CAD build for the part. Positions are in the model's coordinates, mm. Face numbers are marked on the shaded views. A direction names the side the tool comes from. Give positions to 0.01 mm unless a question says otherwise; leave off trailing zeros. Write each loop counter-clockwise with the first axis right and the second up, starting at its lowest first coordinate (ties: lowest second). Pieces come first, ordered by that corner, then holes. Notation, with made-up numbers: M 43,9 L 50,9 A27 cw 50,38 Z; hole C 78,23.25 d8. An arc over 180 degrees is marked long. One line per question, with ' | ' between items. Start each with the question number.
1. Cut at B-B, the plane z = -9.75. Write the cut outline in (x, y), then the cut area to 3 significant figures.
2. Wall check: L1, parallel to X at y = 1, z = 6.5; L2, parallel to Y at x = 7.5, z = 10.5; L3, parallel to Z at x = 11, y = 0.9. Give the ranges that are in metal, low to high.
3. Cut at C-C, the plane y = 1.55. Write the cut outline in (x, z), then the cut area to 3 significant figures.
4. Flat gauge pins, fed straight in: pin 1 (0.6 mm diameter, centred on x = 11, y = 1.5, fed in from +Z); pin 2 (5 mm diameter, centred on x = 1.5, z = -0.5, fed in from +Y). Where does each tip first touch, or does it go through?
5. Cut at D-D, the plane x = -8. Write the cut outline in (y, z).
6. Which spindle directions (+Z, -Z, +X, -X, +Y, -Y) get a long thin tool onto all of the face, cutting with end or side? Do the marked faces 1 and 2. Say none if no direction does.
7. Cut at A-A, the plane x = 11.25. Write the cut outline in (y, z).
```python
from build123d import *

# Parameters (mm, degrees)
SKETCH1_W           = 26
SKETCH1_H           = 24
BOSS_EXTRUDE1_DEPTH = 0.7
SKETCH2_W           = 2
SKETCH2_H           = 22
BOSS_EXTRUDE2_DEPTH = 1.3
CUT_EXTRUDE2_DEPTH  = 0.4
CUT_EXTRUDE3_DEPTH  = 0.4
SKETCH4_W           = 1
SKETCH4_H           = 24
BOSS_EXTRUDE3_DEPTH = 0.7
CUT_EXTRUDE4_DEPTH  = 0.4


with BuildPart() as part:
    # Sketch1 → Boss-Extrude1 (new body)
    with BuildSketch(Plane(origin=(0, 0, 0), x_dir=(1, 0, 0), z_dir=(0, 1, 0))):
        Rectangle(SKETCH1_W, SKETCH1_H)
    extrude(amount=BOSS_EXTRUDE1_DEPTH)

    # Sketch2 → Boss-Extrude2 (add)
    with BuildSketch(Plane(origin=(0, 0.7, 0), x_dir=(1, 0, 0), z_dir=(0, 1, 0))):
        with Locations((11, 0)):
            Rectangle(SKETCH2_W, SKETCH2_H)
    extrude(amount=BOSS_EXTRUDE2_DEPTH)

    # Sketch3 → Cut-Extrude2 (cut)
    with BuildSketch(Plane(origin=(0, 0.7, 0), x_dir=(1, 0, 0), z_dir=(0, 1, 0))):
        with BuildLine():
            Line((-2.366025404, 7.5), (-11.026279442, -7.5))
            ThreePointArc((-11.026279442, -7.5), (-11.026279442, -8.5), (-10.160254038, -9))
            Line((-10.160254038, -9), (7.160254038, -9))
            ThreePointArc((7.160254038, -9), (8.026279442, -8.5), (8.026279442, -7.5))
            Line((8.026279442, -7.5), (-0.633974596, 7.5))
            ThreePointArc((-0.633974596, 7.5), (-1.5, 8), (-2.366025404, 7.5))
        make_face()
        Polygon((7.160254038, -8), (-1.5, 7), (-10.160254038, -8), align=None, mode=Mode.SUBTRACT)
    extrude(amount=-CUT_EXTRUDE2_DEPTH, mode=Mode.SUBTRACT)

    # Sketch5 → Cut-Extrude3 (cut)
    with BuildSketch(Plane(origin=(0, 0.7, 0), x_dir=(1, 0, 0), z_dir=(0, 1, 0))):
        with BuildLine():
            Line((-4.151650429, -6.00520382), (-2.369048338, -4.222601728))
            ThreePointArc((-2.369048338, -4.222601728), (-2.33335535, -4.247204418), (-2.296966313, -4.270765398))
            Line((-2.296966313, -4.270765398), (-2.756186431, -5.379420837))
            Line((-2.756186431, -5.379420837), (-2.294246665, -5.570762553))
            Line((-2.294246665, -5.570762553), (-1.835026546, -4.462107114))
            ThreePointArc((-1.835026546, -4.462107114), (-1.792635483, -4.471177921), (-1.75, -4.479019946))
            Line((-1.75, -4.479019946), (-1.75, -7))
            Line((-1.75, -7), (-1.25, -7))
            Line((-1.25, -7), (-1.25, -4.479019946))
            ThreePointArc((-1.25, -4.479019946), (-1.207364517, -4.471177921), (-1.164973454, -4.462107114))
            Line((-1.164973454, -4.462107114), (-0.705753335, -5.570762553))
            Line((-0.705753335, -5.570762553), (-0.243813569, -5.379420837))
            Line((-0.243813569, -5.379420837), (-0.703033687, -4.270765398))
            ThreePointArc((-0.703033687, -4.270765398), (-0.66664465, -4.247204418), (-0.630951662, -4.222601728))
            Line((-0.630951662, -4.222601728), (1.151650429, -6.00520382))
            Line((1.151650429, -6.00520382), (1.50520382, -5.651650429))
            Line((1.50520382, -5.651650429), (-0.277398272, -3.869048338))
            ThreePointArc((-0.277398272, -3.869048338), (-0.252795582, -3.83335535), (-0.229234602, -3.796966313))
            Line((-0.229234602, -3.796966313), (0.879420837, -4.256186431))
            Line((0.879420837, -4.256186431), (1.070762553, -3.794246665))
            Line((1.070762553, -3.794246665), (-0.037892886, -3.335026546))
            ThreePointArc((-0.037892886, -3.335026546), (-0.028822079, -3.292635483), (-0.020980054, -3.25))
            Line((-0.020980054, -3.25), (2.5, -3.25))
            Line((2.5, -3.25), (2.5, -2.75))
            Line((2.5, -2.75), (-0.020980054, -2.75))
            ThreePointArc((-0.020980054, -2.75), (-0.028822079, -2.707364517), (-0.037892886, -2.664973454))
            Line((-0.037892886, -2.664973454), (1.070762553, -2.205753335))
            Line((1.070762553, -2.205753335), (0.879420837, -1.743813569))
            Line((0.879420837, -1.743813569), (-0.229234602, -2.203033687))
            ThreePointArc((-0.229234602, -2.203033687), (-0.252795582, -2.16664465), (-0.277398272, -2.130951662))
            Line((-0.277398272, -2.130951662), (1.50520382, -0.348349571))
            Line((1.50520382, -0.348349571), (1.151650429, 0.00520382))
            Line((1.151650429, 0.00520382), (-0.630951662, -1.777398272))
            ThreePointArc((-0.630951662, -1.777398272), (-0.66664465, -1.752795582), (-0.703033687, -1.729234602))
            Line((-0.703033687, -1.729234602), (-0.243813569, -0.620579163))
            Line((-0.243813569, -0.620579163), (-0.705753335, -0.429237447))
            Line((-0.705753335, -0.429237447), (-1.164973454, -1.537892886))
            ThreePointArc((-1.164973454, -1.537892886), (-1.207364517, -1.528822079), (-1.25, -1.520980054))
            Line((-1.25, -1.520980054), (-1.25, 1))
            Line((-1.25, 1), (-1.75, 1))
            Line((-1.75, 1), (-1.75, -1.520980054))
            ThreePointArc((-1.75, -1.520980054), (-1.792635483, -1.528822079), (-1.835026546, -1.537892886))
            Line((-1.835026546, -1.537892886), (-2.294246665, -0.429237447))
            Line((-2.294246665, -0.429237447), (-2.756186431, -0.620579163))
            Line((-2.756186431, -0.620579163), (-2.296966313, -1.729234602))
            ThreePointArc((-2.296966313, -1.729234602), (-2.33335535, -1.752795582), (-2.369048338, -1.777398272))
            Line((-2.369048338, -1.777398272), (-4.151650429, 0.00520382))
            Line((-4.151650429, 0.00520382), (-4.50520382, -0.348349571))
            Line((-4.50520382, -0.348349571), (-2.722601728, -2.130951662))
            ThreePointArc((-2.722601728, -2.130951662), (-2.747204418, -2.16664465), (-2.770765398, -2.203033687))
            Line((-2.770765398, -2.203033687), (-3.879420837, -1.743813569))
            Line((-3.879420837, -1.743813569), (-4.070762553, -2.205753335))
            Line((-4.070762553, -2.205753335), (-2.962107114, -2.664973454))
            ThreePointArc((-2.962107114, -2.664973454), (-2.971177921, -2.707364517), (-2.979019946, -2.75))
            Line((-2.979019946, -2.75), (-5.5, -2.75))
            Line((-5.5, -2.75), (-5.5, -3.25))
            Line((-5.5, -3.25), (-2.979019946, -3.25))
            ThreePointArc((-2.979019946, -3.25), (-2.971177921, -3.292635483), (-2.962107114, -3.335026546))
            Line((-2.962107114, -3.335026546), (-4.070762553, -3.794246665))
            Line((-4.070762553, -3.794246665), (-3.879420837, -4.256186431))
            Line((-3.879420837, -4.256186431), (-2.770765398, -3.796966313))
            ThreePointArc((-2.770765398, -3.796966313), (-2.747204418, -3.83335535), (-2.722601728, -3.869048338))
            Line((-2.722601728, -3.869048338), (-4.50520382, -5.651650429))
            Line((-4.50520382, -5.651650429), (-4.151650429, -6.00520382))
        make_face()
    extrude(amount=-CUT_EXTRUDE3_DEPTH, mode=Mode.SUBTRACT)

    # Sketch4 → Boss-Extrude3 (add)
    with BuildSketch(Plane(origin=(0, 0.7, 0), x_dir=(1, 0, 0), z_dir=(0, 1, 0))):
        with Locations((-13.5, 0)):
            Rectangle(SKETCH4_W, SKETCH4_H)
    extrude(amount=-BOSS_EXTRUDE3_DEPTH)

    # Sketch6 → Cut-Extrude4 (cut)
    with BuildSketch(Plane(origin=(0, 0.7, 0), x_dir=(1, 0, 0), z_dir=(0, 1, 0))):
        Polygon((2.5, -2.75), (4.129165125, -2.75), (4.417840259, -3.25), (2.5, -3.25), align=None)
    extrude(amount=-CUT_EXTRUDE4_DEPTH, mode=Mode.SUBTRACT)


solid = part.part
```
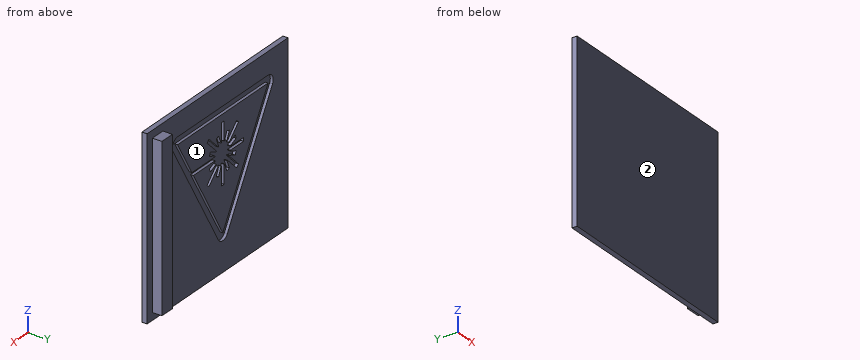
Here are the results:
1) outline: M -14,0 L 13,0 L 13,0.7 L 12,0.7 L 12,2 L 10,2 L 10,0.7 L -14,0.7 Z | area: 21.5 mm^2
2) L1: 10 to 12 | L2: 0 to 0.7 | L3: -11 to 11
3) outline: M 10,-11 L 12,-11 L 12,11 L 10,11 Z | area: 44.0 mm^2
4) pin 1: z = 11 | pin 2: y = 0.7
5) outline: M 0,-12 L 0.7,-12 L 0.7,2.26 L 0.3,2.26 L 0.3,4.26 L 0.7,4.26 L 0.7,8 L 0.3,8 L 0.3,9 L 0.7,9 L 0.7,12 L 0,12 Z
6) face 1: +Z, -Z, -X, +Y | face 2: +Z, -Z, +X, -X, -Y
7) outline: M 0,-12 L 0.7,-12 L 0.7,-11 L 2,-11 L 2,11 L 0.7,11 L 0.7,12 L 0,12 Z
